Check sheet for the drawn part. Datum: minimum x, y, z corner. Units: mm. A direction names the side the tool comes from. Give positions to 0.01 mm unless a question says otherwise; leave off trailing zeros. Write each loop counter-clockwise with the first axis right and the second up, starting at its lowest first coordinate (ties: lowest second). Pieces come first, ordered by that corner, then holes.
(1) Cross-section at A-A (x = 53.5). Record the boundary of the cut face in (y, z) (1 decimal), and give its area (3 significant figures).
(2) Cross-section at B-B (y = 14.5). Record the boundary of the cut face in (x, z).
(3) Tool access check on the marked faces 5 and 6. Record the directions out of +Z, -Z, +X, -X, +Y, -Y that give a thin tool (end or side, any length) a straight path to the whole face; none if there is none.
(4) Depth check by flat-ended pin: P1, Ø3, axis at x = 21.5, z = 30, coming from the -Y side; P2, Ø9.5, axis at x = 12, y = 13.208, coming from the -Z side; P3, Ø12, axis at y = 22.5, z = 12.5, coming from the -X side (1 decimal). Enter the tip coordinate at first touch or a pass-through.
(5) Cross-section at D-D (z = 25). Record the boundary of the cut face in (x, y).
(6) Thickness scan on line 1 along Y through (x, z) = (43, 10.5); line 2 along Z through (x, y) = (53, 19.25); line 3 along Z through (x, y) = (34.5, 3) (1 decimal). Record the ranges inside material, lowest first.
(7) Mould release check, pull along Y, two halves, no side actions. Record for the marked faces 1, 2, 3 and 4: +Y half, -Y half, draft (parallel to the pull), parting line (faces both ways), or undercut.
(8) Cross-section at C-C (x = 12). Record the boundary of the cut face in (y, z).
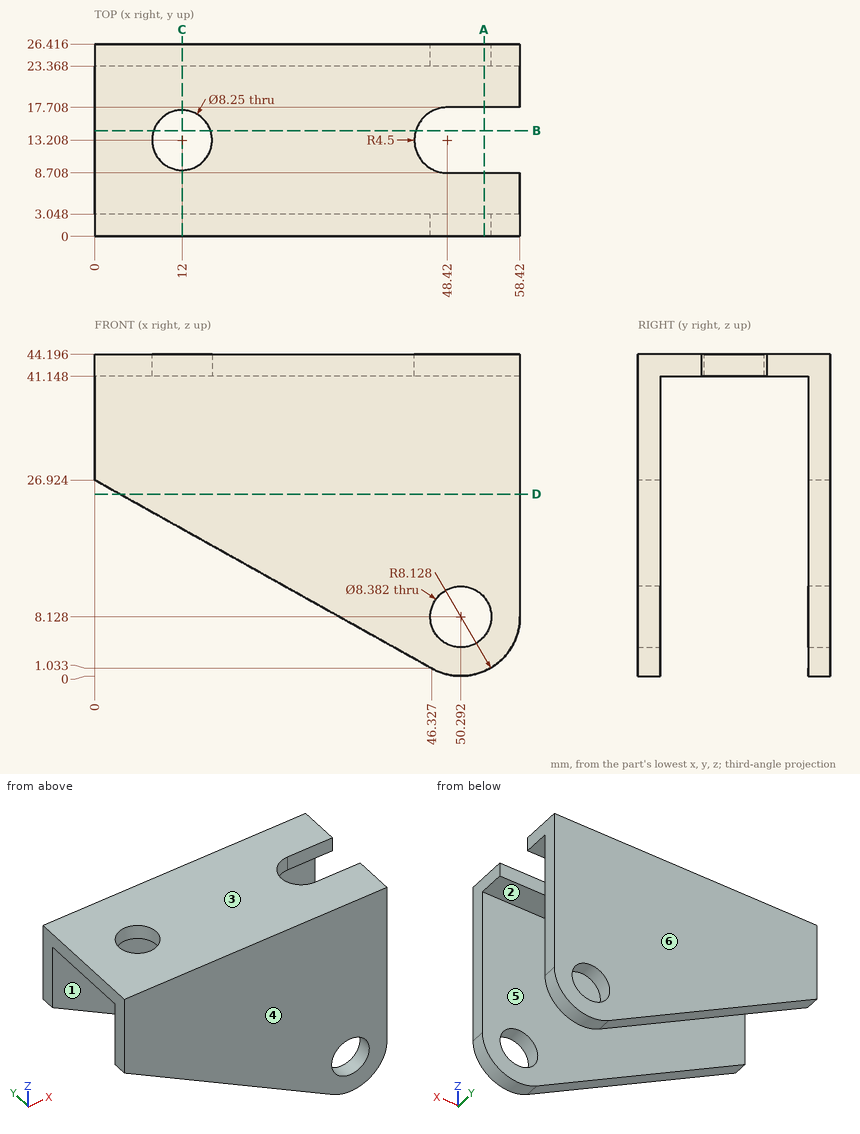
Reply:
1. outline: (0, 0.7) - (3, 0.7) - (3, 5.4) - (0, 5.4) - close; (0, 10.8) - (3, 10.8) - (3, 41.1) - (8.7, 41.1) - (8.7, 44.2) - (0, 44.2) - close; (17.7, 41.1) - (23.4, 41.1) - (23.4, 10.8) - (26.4, 10.8) - (26.4, 44.2) - (17.7, 44.2) - close; (23.4, 0.7) - (26.4, 0.7) - (26.4, 5.4) - (23.4, 5.4) - close
1. area: 267 mm2
2. outline: (0, 41.15) - (8.08, 41.15) - (8.08, 44.2) - (0, 44.2) - close; (15.92, 41.15) - (44.11, 41.15) - (44.11, 44.2) - (15.92, 44.2) - close
3. face 5: -Z, +X, -X
3. face 6: +Z, -Z, +X, -X, +Y
4. P1: stops at y = 0
4. P2: stops at z = 41.15
4. P3: stops at x = 15.2
5. outline: (3.44, 0) - (58.42, 0) - (58.42, 3.05) - (3.44, 3.05) - close; (3.44, 23.37) - (58.42, 23.37) - (58.42, 26.42) - (3.44, 26.42) - close
6. line 1: y = 0 to 3.05, 23.37 to 26.42
6. line 2: z = 41.15 to 44.2
6. line 3: z = 7.6 to 44.2
7. face 1: undercut
7. face 2: undercut
7. face 3: draft
7. face 4: -Y half
8. outline: (0, 20.22) - (3.05, 20.22) - (3.05, 41.15) - (9.08, 41.15) - (9.08, 44.2) - (0, 44.2) - close; (17.33, 41.15) - (23.37, 41.15) - (23.37, 20.22) - (26.42, 20.22) - (26.42, 44.2) - (17.33, 44.2) - close
